from build123d import *

# Parameters (mm, degrees)
ESQUISSE1_W             = 20.75
ESQUISSE1_H             = 14.7
BOSS_EXTRU_1_DEPTH      = 2.1
ESQUISSE2_W             = 18.4
ESQUISSE2_H             = 12.25
BOSS_EXTRU_2_DEPTH      = 14
ESQUISSE3_W             = 0.8
ESQUISSE3_H             = 4.8
BOSS_EXTRU_3_DEPTH      = 6.57
ESQUISSE4_W             = 14.99
ESQUISSE4_H             = 9.5
BOSS_EXTRU_4_DEPTH      = 2
ENL_V_MAT_EXTRU_1_REACH = 29.712


with BuildPart() as part:
    # Esquisse1 → Boss.-Extru.1 (new body)
    with BuildSketch(Plane.XY):
        Rectangle(ESQUISSE1_W, ESQUISSE1_H)
    extrude(amount=BOSS_EXTRU_1_DEPTH)

    # Esquisse2 → Boss.-Extru.2 (add)
    with BuildSketch(Plane.XY.offset(2.1)):
        Rectangle(ESQUISSE2_W, ESQUISSE2_H)
    extrude(amount=BOSS_EXTRU_2_DEPTH)

    # Esquisse3 → Boss.-Extru.3 (add)
    with BuildSketch(Plane.XY.offset(16.1)):
        with Locations((-0.366571113, 0)):
            Rectangle(ESQUISSE3_W, ESQUISSE3_H)
        with Locations((6.633428887, 0)):
            Rectangle(ESQUISSE3_W, ESQUISSE3_H)
        with Locations((-7.366571113, 0)):
            Rectangle(ESQUISSE3_W, ESQUISSE3_H)
    extrude(amount=BOSS_EXTRU_3_DEPTH)

    # Esquisse4 → Boss.-Extru.4 (add)
    with BuildSketch(Plane(origin=(0, 0, 0), x_dir=(-1, 0, 0), z_dir=(0, 0, -1))):
        Rectangle(ESQUISSE4_W, ESQUISSE4_H)
    extrude(amount=BOSS_EXTRU_4_DEPTH)

    # Esquisse5 → Enlèv. mat.-Extru.1 (cut, up to next)
    with BuildSketch(Plane(origin=(0, 4.75, 0), x_dir=(1, 0, 0), z_dir=(0, 1, 0)), mode=Mode.PRIVATE) as enl_v_mat_extru_1_sk1:
        with BuildLine():
            Line((-7.495, 2), (7.495, 2))
            ThreePointArc((7.495, 2), (0, 0.856909001), (-7.495, 2))
        make_face()
    enl_v_mat_extru_1_tool1 = extrude(enl_v_mat_extru_1_sk1.sketch, amount=-ENL_V_MAT_EXTRU_1_REACH, mode=Mode.PRIVATE) & part.part
    add(enl_v_mat_extru_1_tool1.solids().sort_by_distance((0, 4.75, -1.541861))[0], mode=Mode.SUBTRACT)


solid = part.part
Build history of the part. All positions in model axes, mm. A direction names the side the tool comes from. Round coordinates to 2 decimals unless told otherwise and drop trailing zeros. Loops run counter-clockwise (first coordinate to the right, second up) from the corner with the lowest first, then second, coordinate; pieces in that order, holes last. Notation, with made-up numbers: (-10.5, 76) -> (44.5, 76) arc R23 cw to (44.5, 97) -> close; hole circle Ø9 at (-36.75, 79). An arc over 180 degrees is marked (long way). One line per item, written item: value. Start each with the question number.
Q1. Cut at C-C on x = 8.25. List the corners of the cut face in (y, z) (3 decimals), plus the area to 3 significant figures.
Q2. Drop flat-ended pins along their axis: pin 1 Ø5.5 at (y, z) = (0, 20) entering from -X; pin 2 Ø2 at (x, z) = (5.5, 16) entering from -Y (3 decimals); pin 3 Ø0.6 at (x, z) = (-0.5, 19) entering from +Y; pin 4 Ø12 at (x, z) = (4, 5) entering from +Y. Give the stop position or say it passes through.
Q3. Cut at B-B on y = -5.25. List the corners of the cut face in (x, z) (3 decimals).
Q4. Probe line 1 along Z through (x, y) = (6.5, -5.25); line 2 along Y through (x, z) = (8.75, 3.5) (3 decimals); line 3 along X through (y, z) = (4.25, 11.25). List the from-to ranges inside material, lowest first.
Q5. Cut at D-D on z = 7.5. List the corners of the cut face in (x, y) (3 decimals), plus the area to 3 significant figures.
Q6. 3-axis set-ups, long thin cutter, end or side, ignore diameter. For faces 4 (the face through (7.033, 0, 19)), 5 (the face through (-7.495, 0, -1)), 6 (the face through (0, 6.125, 9)), 7 (the face through (6.6, -2.4, 19.3)): which of +Z, -Z, +X, -X, +Y, -Y reach the whole face in a straight line?
Q7. Two-plate mould, pull along X, no slides. Class faces 1 (the face through (0.033, 0, 19)), 2 (the face through (7.495, 0, -1)), 3 (the face through (-7.4, 2.4, 19.3)): released by +X, released by -X, zero draft, split by the parting line, or undercut.
Q8. Cut at A-A on z = 19.75. List the corners of the cut face in (x, y).
Computed:
1. outline: (-7.35, 0) -> (7.35, 0) -> (7.35, 2.1) -> (6.125, 2.1) -> (6.125, 16.1) -> (-6.125, 16.1) -> (-6.125, 2.1) -> (-7.35, 2.1) -> close
1. area: 202 mm²
2. pin 1: x = -7.77
2. pin 2: y = -6.125
2. pin 3: y = 2.4
2. pin 4: y = 7.35
3. outline: (-10.375, 0) -> (10.375, 0) -> (10.375, 2.1) -> (9.2, 2.1) -> (9.2, 16.1) -> (-9.2, 16.1) -> (-9.2, 2.1) -> (-10.375, 2.1) -> close
4. line 1: 0 to 16.1
4. line 2: -6.125 to 6.125
4. line 3: -9.2 to 9.2
5. outline: (-9.2, -6.125) -> (9.2, -6.125) -> (9.2, 6.125) -> (-9.2, 6.125) -> close
5. area: 225 mm²
6. face 4: +Z, +X, +Y, -Y
6. face 5: -Z, -X, +Y, -Y
6. face 6: +Z, +X, -X, +Y
6. face 7: +Z, +X, -X, -Y
7. face 1: undercut
7. face 2: released by +X
7. face 3: zero draft
8. outline: (-7.77, -2.4) -> (-6.97, -2.4) -> (-6.97, 2.4) -> (-7.77, 2.4) -> close; (-0.77, -2.4) -> (0.03, -2.4) -> (0.03, 2.4) -> (-0.77, 2.4) -> close; (6.23, -2.4) -> (7.03, -2.4) -> (7.03, 2.4) -> (6.23, 2.4) -> close
